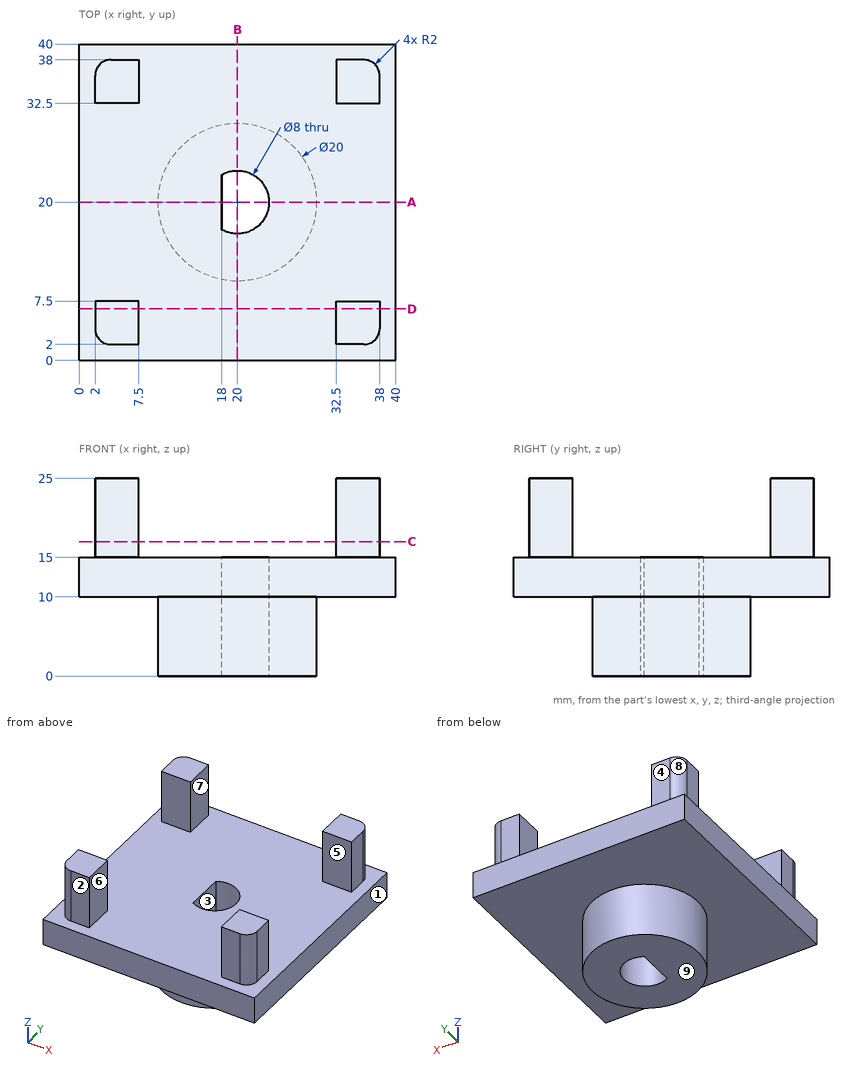
Job drawing, mm, ordinate dimensions from the low corner. One solid piece. A direction names the side the tool comes from. Coordinates: 2 decimals unless noted, no trailing zeros. Write each loop counter-clockwise with the first axis right and the second up, starting at its lowest first coordinate (ties: lowest second). Pieces come first, ordered by that corner, then holes. Notation, with made-up numbers: M 33.5,83 L 89.5,83 A15 ccw 89.5,97 Z; hole C 68.5,81.5 d8. An arc over 180 degrees is marked long. Answer as a JSON object with one key per item and string values. Group by question number.
1) Pin check, flat tips, straight feed: pin 1 Ø1 at (y, z) = (25, 17) entering from -X (3 decimals); pin 2 Ø1.6 at (x, z) = (3.5, 20) entering from -Y; pin 3 Ø3 at (x, z) = (34, 20) entering from +Y; pin 4 Ø1 at (x, y) = (6, 9.5) entering from -Z. Stop position of each tip, or through.
2) Mould opens along X. For the marked faces 6, 7, 8 and 9 say: +X half, -X half, draft (parallel to the pull), parting line (faces both ways), or undercut.
3) Saw through at B-B (x = 20). Write the cut outline in (y, z), plus the area to 3 significant figures.
4) Saw through at D-D (y = 6.5). Write the cut outline in (x, z), plus the area to 3 significant figures.
5) Tool access for the marked faces 1, 2, 3, 4 and 5: list every direction of +Z, -Z, +X, -X, +Y, -Y with a clear straight run to the whole face (end or side of a thin tool).
6) Saw through at A-A (y = 20). Write the cut outline in (x, z).
7) Saw through at C-C (z = 17). Write the cut outline in (x, y).
8) Wall check: line 1 (Y direction, x = 20, z = 11.25); line 2 (X direction, y = 20, z = 5); line 3 (Y direction, x = 20, z = 6.75). Give the ranges that are in metal, low to high. Write a range as from..to.
Values follow:
{
 "1": {"pin 1": "passes through", "pin 2": "stops at y = 2", "pin 3": "stops at y = 38", "pin 4": "stops at z = 10"},
 "2": {"face 6": "undercut", "face 7": "undercut", "face 8": "-X half", "face 9": "draft"},
 "3": {"outline": "M 0,10 L 10,10 L 10,0 L 16,0 L 16,15 L 0,15 Z; M 24,0 L 30,0 L 30,10 L 40,10 L 40,15 L 24,15 Z", "area": "280 mm2"},
 "4": {"outline": "M 0,10 L 40,10 L 40,15 L 38,15 L 38,25 L 32.5,25 L 32.5,15 L 7.5,15 L 7.5,25 L 2,25 L 2,15 L 0,15 Z", "area": "310 mm2"},
 "5": {"face 1": "+Z, -Z, +X, +Y, -Y", "face 2": "+Z, +X, -X, -Y", "face 3": "+Z, -Z", "face 4": "+Z, +X, -X, +Y", "face 5": "+Z, +X, -X"},
 "6": {"outline": "M 0,10 L 10,10 L 10,0 L 18,0 L 18,15 L 0,15 Z; M 24,0 L 30,0 L 30,10 L 40,10 L 40,15 L 24,15 Z"},
 "7": {"outline": "M 2,4 A2 ccw 4,2 L 7.5,2 L 7.5,7.5 L 2,7.5 Z; M 2,32.5 L 7.5,32.5 L 7.5,38 L 4,38 A2 ccw 2,36 Z; M 32.5,2 L 36,2 A2 ccw 38,4 L 38,7.5 L 32.5,7.5 Z; M 32.5,32.5 L 38,32.5 L 38,36 A2 ccw 36,38 L 32.5,38 Z"},
 "8": {"line 1": "y = 0..16, 24..40", "line 2": "x = 10..18, 24..30", "line 3": "y = 10..16, 24..30"}
}
